Solid Edge part; units mm, degrees
sketch "Sketch1" plane through (0, 0, 0) normal (0, 0, 1) x (1, 0, 0)
  line L0 (40, -25) -> (40, 30)
  line L1 (40, 30) -> (-44, 30)
  line L2 (-44, 30) -> (-44, -25)
  line L3 (-44, -25) -> (40, -25)
extrude "Protrusion1" add sketch "Sketch1" along normal blind 2
sketch "Sketch2" plane through (0, 0, 0) normal (0, 0, 1) x (1, 0, 0)
  line L0 (-44, 28) -> (-27, 28)
  line L1 (-27, 28) -> (-27, 30)
  line L2 (-27, 30) -> (-44, 30)
  line L3 (-44, 30) -> (-44, 28)
extrude "ExtrudedCutout_1" cut sketch "Sketch2" along normal blind 2
sketch "Sketch3" plane through (0, 0, 0) normal (0, 0, 1) x (1, 0, 0)
  line L0 (-17, 28) -> (13, 28)
  line L1 (13, 28) -> (13, 30)
  line L2 (13, 30) -> (-17, 30)
  line L3 (-17, 30) -> (-17, 28)
extrude "ExtrudedCutout_2" cut sketch "Sketch3" along normal blind 2
sketch "Sketch4" plane through (0, 0, 0) normal (0, 0, 1) x (1, 0, 0)
  line L0 (23, 28) -> (40, 28)
  line L1 (40, 28) -> (40, 30)
  line L2 (40, 30) -> (23, 30)
  line L3 (23, 30) -> (23, 28)
extrude "ExtrudedCutout_3" cut sketch "Sketch4" along normal blind 2
sketch "Sketch5" plane through (0, 0, 0) normal (0, 0, 1) x (1, 0, 0)
  line L0 (38, -2.5) -> (38, 7.5)
  line L1 (38, 7.5) -> (36, 7.5)
  line L2 (36, 7.5) -> (36, -2.5)
  line L3 (36, -2.5) -> (38, -2.5)
extrude "ExtrudedCutout_4" cut sketch "Sketch5" along normal blind 2
sketch "Sketch6" plane through (0, 0, 0) normal (0, 0, 1) x (1, 0, 0)
  line L0 (40, -23) -> (23, -23)
  line L1 (23, -23) -> (23, -25)
  line L2 (23, -25) -> (40, -25)
  line L3 (40, -25) -> (40, -23)
extrude "ExtrudedCutout_5" cut sketch "Sketch6" along normal blind 2
sketch "Sketch7" plane through (0, 0, 0) normal (0, 0, 1) x (1, 0, 0)
  line L0 (13, -23) -> (-17, -23)
  line L1 (-17, -23) -> (-17, -25)
  line L2 (-17, -25) -> (13, -25)
  line L3 (13, -25) -> (13, -23)
extrude "ExtrudedCutout_6" cut sketch "Sketch7" along normal blind 2
sketch "Sketch8" plane through (0, 0, 0) normal (0, 0, 1) x (1, 0, 0)
  line L0 (-27, -23) -> (-44, -23)
  line L1 (-44, -23) -> (-44, -25)
  line L2 (-44, -25) -> (-27, -25)
  line L3 (-27, -25) -> (-27, -23)
extrude "ExtrudedCutout_7" cut sketch "Sketch8" along normal blind 2
sketch "Sketch9" plane through (0, 0, 0) normal (0, 0, 1) x (1, 0, 0)
  line L0 (-40, -2.5) -> (-40, 7.5)
  line L1 (-40, 7.5) -> (-42, 7.5)
  line L2 (-42, 7.5) -> (-42, -2.5)
  line L3 (-42, -2.5) -> (-40, -2.5)
extrude "ExtrudedCutout_8" cut sketch "Sketch9" along normal blind 2
sketch "Sketch10" plane through (0, 0, 0) normal (0, 0, 1) x (1, 0, 0)
  circle A0 centre (-35.6965, 23.0215) radius 1.8
extrude "Cutout1" cut sketch "Sketch10" along normal blind 2
sketch "Sketch11" plane through (0, 0, 0) normal (0, 0, 1) x (1, 0, 0)
  circle A0 centre (5.3589, 23.016) radius 1.8
extrude "ExtrudedCutout_10" cut sketch "Sketch11" along normal blind 2
sketch "Sketch12" plane through (0, 0, 0) normal (0, 0, 1) x (1, 0, 0)
  circle A0 centre (-35.7266, -17.9943) radius 1.8
extrude "ExtrudedCutout_11" cut sketch "Sketch12" along normal blind 2
sketch "Sketch13" plane through (0, 0, 0) normal (0, 0, 1) x (1, 0, 0)
  circle A0 centre (5.346, -18.0319) radius 1.8
extrude "ExtrudedCutout_12" cut sketch "Sketch13" along normal blind 2
sketch "Sketch14" plane through (0, 0, 0) normal (0, 0, 1) x (1, 0, 0)
  circle A0 centre (-24.2914, 11.6184) radius 1
  circle A1 centre (-19.6326, 6.9596) radius 1
  circle A2 centre (-15.1715, 2.4985) radius 1
  circle A3 centre (-10.7104, 6.9596) radius 1
  circle A4 centre (-6.0516, 11.6184) radius 1
  circle A5 centre (-10.7104, -1.9626) radius 1
  circle A6 centre (-6.0516, -6.6214) radius 1
  circle A7 centre (-19.6326, -1.9626) radius 1
  circle A8 centre (-24.2914, -6.6214) radius 1
extrude "ExtrudedCutout_13" cut sketch "Sketch14" along normal blind 2
properties material "Acrylic, high impact grade"
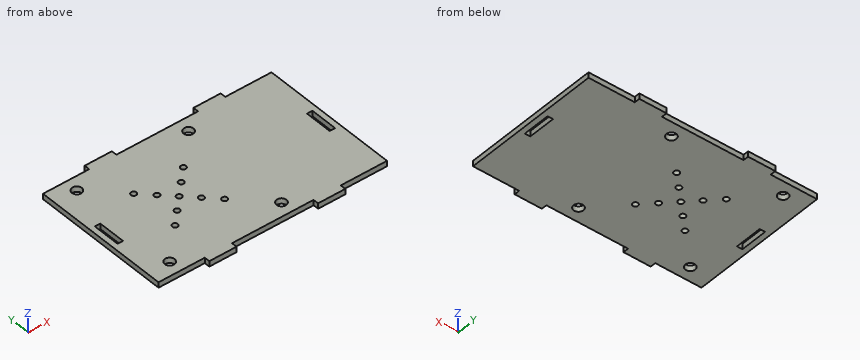
The listing builds one solid part. Answer for the finished solid, in the listing's coordinates (mm). Give positions to 0.01 mm unless a question says otherwise; leave off trailing zeros. Order: outer loops, then holes, each group sorted by start corner. A loop starts at its lowest first (then second) coordinate and runs counter-clockwise, first axis right, second up. Notation, with made-up numbers: (-23.5, 70) - (31.5, 70) arc R19 cw to (31.5, 74) - close; hole circle Ø1 at (89.25, 5.25). An arc over 180 degrees is marked (long way). Answer in a Markdown table with one row per item. Add a question column.
Q1. Given P1, Ø1, axis at y = 29.5, z = 1, coming from the -X side; P2, Ø1, axis at x = -33.5, z = 1.5, coming from the +Y side; P3, Ø1, axis at x = 35.5, z = 0.5, coming from the -Y side, each flat-ended and moving along its own axis, determine where each tip first touches the part or whether it passes through.
Q2. The part is cut by section A-A (x = 5). Determine the outline of the cut face in (y, z), then the cut area to 3 significant figures.
Q3. The part is cut by section C-C (z = 0.85). Give the number of separate pieces and of enclosed holes in the cut face, then the cut area to 4 significant figures.
Q4. The part is cut by section B-B (x = 30.5). Determine the outline of the cut face in (y, z).
Q5. Find the intervals of material crossed by line 1 along X through (y, z) = (0, 1.3); line 2 along X through (y, z) = (-2, 1.05); line 3 along X through (y, z) = (24, 1.8), in increasing order. Write a range as [from, to].
Determined:
| question | item | result |
|---|---|---|
| 1 | P1 | stops at x = -27 |
| 1 | P2 | stops at y = 28 |
| 1 | P3 | stops at y = -23 |
| 2 | outline | (-23, 0) - (-19.8, 0) - (-19.8, 2) - (-23, 2) - close; (-16.27, 0) - (21.25, 0) - (21.25, 2) - (-16.27, 2) - close; (24.78, 0) - (28, 0) - (28, 2) - (24.78, 2) - close |
| 2 | area | 87.9 mm² |
| 3 | separate pieces | 1 |
| 3 | enclosed holes | 15 |
| 3 | area | 4,255 mm² |
| 4 | outline | (-23, 0) - (28, 0) - (28, 2) - (-23, 2) - close |
| 5 | line 1 | x = [-44, -42], [-40, 36], [38, 40] |
| 5 | line 2 | x = [-44, -42], [-40, -20.63], [-18.63, -11.71], [-9.71, 36], [38, 40] |
| 5 | line 3 | x = [-44, -37.21], [-34.19, 3.85], [6.87, 40] |
